```python
from build123d import *

# Parameters (mm, degrees)
F0_R     = 12.7
F1_DEPTH = 25.4
F2_R     = 12.7
F3_DEPTH = 254
F4_R     = 5.08
F5_R     = 10.16
F6_R     = 5.08


with BuildPart() as f1:
    # F0 (on Top) → F1 (new body)
    with BuildSketch(Plane.XY):
        with BuildLine():
            Line((26.491852, 17.019746), (26.491852, 118.097939))
            ThreePointArc((26.491852, 118.097939), (-6.261039, 150.85083), (-39.013931, 118.097939))
            Line((-39.013931, 118.097939), (-39.013931, 37.074262))
            ThreePointArc((-39.013931, 37.074262), (-24.833246, 31.20043), (-18.959414, 17.019746))
            Line((-18.959414, 17.019746), (26.491852, 17.019746))
        make_face()
        with Locations((-6.261039, 118.097939)):
            Circle(F0_R, mode=Mode.SUBTRACT)
    extrude(amount=F1_DEPTH)

    # F2 (on face) → F3 (join)
    with BuildSketch(Plane.XY.offset(25.4)):
        with Locations((-6.261039, 118.097939)):
            Circle(F2_R)
    extrude(amount=-F3_DEPTH)

    # F4
    f4_edges = [f1.edges().sort_by_distance(p)[0] for p in [
        (-18.961039, 118.097939, -228.6),
    ]]
    fillet(f4_edges, radius=F4_R)

    # F5
    f5_edges = [f1.edges().sort_by_distance(p)[0] for p in [
        (26.491852, 17.019746, 12.7),
        (-18.959414, 17.019746, 12.7),
        (-39.013931, 37.074262, 12.7),
    ]]
    fillet(f5_edges, radius=F5_R)

    # F6
    f6_edges = [f1.edges().sort_by_distance(p)[0] for p in [
        (-39.013931, 81.786381, 25.4),
        (-39.013931, 81.786381, 0),
    ]]
    fillet(f6_edges, radius=F6_R)


solid = f1.part
```
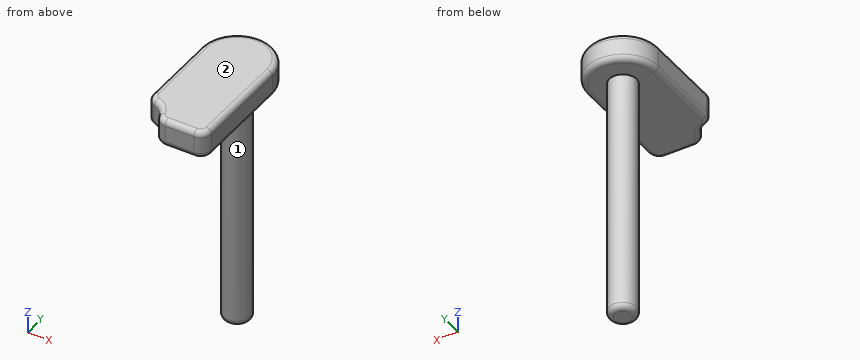
Build history of the part. All positions in model axes, mm. Face numbers are marked on the shaded views. A direction names the side the tool comes from. Coordinates: 2 decimals unless noted, no trailing zeros. Order: outer loops, then holes, each group sorted by start corner. A loop starts at its lowest first (then second) coordinate and runs counter-clockwise, first axis right, second up. Notation, with made-up numbers: (36, -33.5) -> (72, -33.5) arc R24 ccw to (72, 4.5) -> close; hole circle Ø11 at (75.5, 67.25). An arc over 180 degrees is marked (long way). Answer in a Markdown table with one row per item. Add a question column.
Q1. Band-saw the part on A-A, the plane y = 94. List the corners of the cut face in (x, z), then the cut area to 3 significant figures.
Q2. Which spindle directions (+Z, -Z, +X, -X, +Y, -Y) get a long thin tool onto all of the face, cutting with end or side? Do the marked faces 1 and 2. Say none if no direction does.
Q3. Band-saw the part on B-B, the plane z = 9. List the corners of the cut face in (x, y).
Q4. Band-saw the part on C-C, the plane z = -109. List the corners of the cut face in (x, y), then the cut area to 3 significant figures.
Q5. Wall check: line 1 along Z through (x, y) = (20, 108.5); line 2 along Y through (x, z) = (-9.5, -102); line 3 along Y through (x, z) = (2.5, -46). Give the ranges that are in metal, low to high. Write a range as [from, to].
Q6. Drop flat-ended pins along their axis: pin 1 (1 mm diameter, centred on y = 132.5, z = -109.5, fed in from -X); pin 2 (5 mm diameter, centred on x = 5, z = -89.5, fed in from +Y); pin 3 (2 mm diameter, centred on x = 15.5, y = 33.5, fed in from -Z); pin 4 (3 mm diameter, centred on y = 106.5, z = -87.5, fed in from +X). Give the stop position or say it passes through.
Answers follow:
| question | item | result |
|---|---|---|
| 1 | outline | (-39.01, 5.08) arc R5.08 ccw to (-33.93, 0) -> (21.41, 0) arc R5.08 ccw to (26.49, 5.08) -> (26.49, 20.32) arc R5.08 ccw to (21.41, 25.4) -> (-33.93, 25.4) arc R5.08 ccw to (-39.01, 20.32) -> close |
| 1 | area | 1,640 mm^2 |
| 2 | face 1 | -Z |
| 2 | face 2 | +Z, +X, -X, +Y, -Y |
| 3 | outline | (-39.01, 45.47) arc R10.16 ccw to (-32.27, 35.91) arc R20.05 cw to (-20.13, 23.76) arc R10.16 ccw to (-10.56, 17.02) -> (16.33, 17.02) arc R10.16 ccw to (26.49, 27.18) -> (26.49, 118.1) arc R32.75 ccw to (-39.01, 118.1) -> close |
| 4 | outline | circle Ø25.4 at (-6.26, 118.1) |
| 4 | area | 507 mm^2 |
| 5 | line 1 | [0, 25.4] |
| 5 | line 2 | [105.82, 130.38] |
| 5 | line 3 | [108.9, 127.29] |
| 6 | pin 1 | through |
| 6 | pin 2 | y = 127.29 |
| 6 | pin 3 | z = 0 |
| 6 | pin 4 | x = 1.44 |
